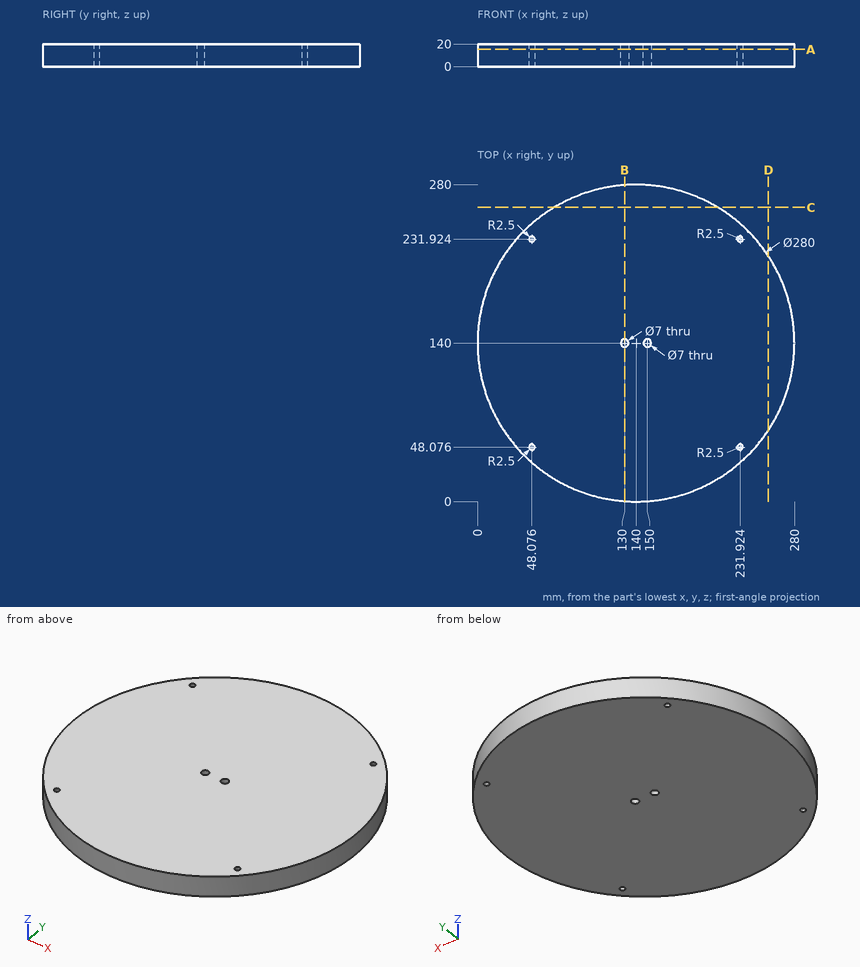
Input: dimensioned drawing with shaded views. Units: mm. Origin: part minimum x, y, z. Coordinates: 2 decimals unless noted, no trailing zeros. Loops run counter-clockwise (first coordinate to the right, second up) from the corner with the lowest first, then second, coordinate; pieces in that order, holes last. Notation, with made-up numbers: M 43.5,-11 L 53.5,-11 A19 ccw 53.5,20 Z; hole C 53,-12.75 d1. An arc over 180 degrees is marked long. One line per item, written item: value. Start each with the question number.
1) Pin query (flat end, axial travel): P1, Ø4, axis at x = 150, y = 140, coming from the -Z side; P2, Ø2, axis at x = 167, z = 8.5, coming from the +Y side; P3, Ø1.5, axis at y = 246, z = 8, coming from the +X side; P4, Ø3, axis at x = 165.5, z = 8, coming from the -Y side. Return the tip coordinate at first contact, or that it passes through.
2) Material intervals for L1, parallel to Y at x = 150, z = 16; L2, parallel to Y at x = 39, z = 7.5; L3, parallel to X at y = 225.5, z = 4.75, sorted ascending. Write a range as from..to.
3) Cut plane C-C (y = 260). Return loops of the section in (x, z), then the cut area to 3 significant figures.
4) Cut plane D-D (x = 257). Return loops of the section in (y, z).
5) Cut plane B-B (x = 130). Return loops of the section in (y, z).
6) Cut plane A-A (z = 15.25). Return loops of the section in (x, y).
Evaluation:
1. P1: through
1. P2: y = 277.56
1. P3: x = 232.32
1. P4: y = 2.07
2. L1: 0.36..136.5, 143.5..279.64
2. L2: 43.05..236.95
2. L3: 29.14..250.86
3. outline: M 67.89,0 L 212.11,0 L 212.11,20 L 67.89,20 Z
3. area: 2,880 mm^2
4. outline: M 63.12,0 L 216.88,0 L 216.88,20 L 63.12,20 Z
5. outline: M 0.36,0 L 136.5,0 L 136.5,20 L 0.36,20 Z; M 143.5,0 L 279.64,0 L 279.64,20 L 143.5,20 Z
6. outline: C 140,140 d280; hole M 46.33,49.86 A2.5 ccw long 49.86,46.33 A2.5 ccw 50.58,48.08 A2.5 ccw 49.84,49.84 A2.5 ccw Z; hole M 46.33,230.14 A2.5 ccw 49.84,230.16 A2.5 ccw 50.58,231.92 A2.5 ccw 49.86,233.67 A2.5 ccw long Z; hole C 130,140 d7; hole C 150,140 d7; hole M 230.14,46.33 A2.5 ccw 234.42,48.08 A2.5 ccw 233.67,49.86 A2.5 ccw 230.16,49.84 A2.5 ccw Z; hole M 230.14,233.67 A2.5 ccw 230.16,230.16 A2.5 ccw 233.67,230.14 A2.5 ccw 234.42,231.92 A2.5 ccw Z
